from build123d import *

# Parameters (mm, degrees)
PROFILE_SKETCH_W               = 6
PROFILE_SKETCH_H               = 1
PROFILE_EXTRUDE_DEPTH          = 40
FIDUCIAL_CUT_DEPTH             = 44.409509652
FIDUCIAL_1_INDICATOR_SKETCH_W  = 2
FIDUCIAL_1_INDICATOR_SKETCH_H  = 2
FIDUCIAL_1_INDICATOR_CUT_DEPTH = 44.409509652


with BuildPart() as part:
    # Profile Sketch → Profile Extrude (new body)
    with BuildSketch(Plane(origin=(-13.83405858, 0, -105.75669297), x_dir=(-1, 0, 0), z_dir=(0, 1, 0))):
        with Locations((0, 0.5)):
            Rectangle(PROFILE_SKETCH_W, PROFILE_SKETCH_H)
    extrude(amount=PROFILE_EXTRUDE_DEPTH)

    # Fiducial Sketch → Fiducial Cut (cut, through all)
    with BuildSketch(Plane.XY.offset(-104.75669297)):
        Polygon((-12.669845017, 2), (-14.08405858, 3.414213562), (-15.498272142, 2), (-14.08405858, 0.585786438), align=None)
    fiducial_cut = extrude(amount=-FIDUCIAL_CUT_DEPTH, mode=Mode.SUBTRACT)

    # Fiducial Mirror: Fiducial Cut across plane
    add(fiducial_cut.mirror(Plane(origin=(0, 20, 0), x_dir=(0, 0, 1), z_dir=(0, -1, 0))), mode=Mode.SUBTRACT)

    # Fiducial 1 Indicator Sketch → Fiducial 1 Indicator Cut (cut, through all)
    with BuildSketch(Plane.XY.offset(-104.75669297)):
        with Locations((-14.08405858, 6)):
            Rectangle(FIDUCIAL_1_INDICATOR_SKETCH_W, FIDUCIAL_1_INDICATOR_SKETCH_H)
    extrude(amount=-FIDUCIAL_1_INDICATOR_CUT_DEPTH, mode=Mode.SUBTRACT)


solid = part.part
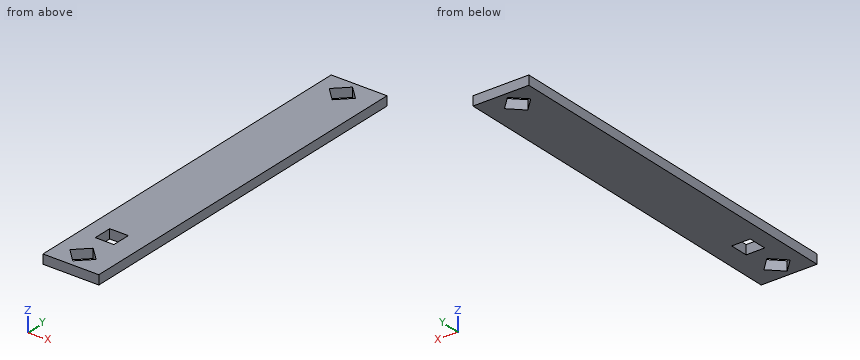
For this review, take the finished solid that the model builds, in its own axes (mm). Give positions to 0.01 mm unless a question says otherwise; leave off trailing zeros. Loops run counter-clockwise (first coordinate to the right, second up) from the corner with the lowest first, then second, coordinate; pieces in that order, holes last. Notation, with made-up numbers: M 69.25,-34 L 76.25,-34 A10 cw 76.25,-30 Z; hole C 41.25,74.5 d7. An arc over 180 degrees is marked long. Answer as a JSON object with one key per item and string values. Group by question number.
Q1. Insertion check: P1, Ø0.5, axis at x = -14, z = -105.5, coming from the -Y side. The pin has a flat end and moves straight along its axis. Give the tip position at first contact, or say it passes through.
Q2. For probe 1 along Y at (x, z) = (-14.9, -105.4); probe 2 along Y at (x, z) = (-13.6, -105.5); probe 3 along X at (y, z) = (37.5, -105.45), list the stretches that pass through material, from the lowest coordinate up. Write a range as [from, to].
Q3. Add section A-A on z = -105.2. Give the boundary of the cut face in (x, y), and give its area (3 significant figures).
Q4. Add section B-B on x = -13.7. Give the boundary of the cut face in (y, z).
Checked values:
{
 "1": {"P1": "y = 0"},
 "2": {"probe 1": "[0, 1.4], [2.6, 5], [7, 37.4], [38.6, 40]", "probe 2": "[0, 1.07], [2.93, 5], [7, 37.07], [38.93, 40]", "probe 3": "[-16.83, -15], [-13.17, -10.83]"},
 "3": {"outline": "M -16.83,0 L -10.83,0 L -10.83,40 L -16.83,40 Z; hole M -15.5,2 L -14.08,0.59 L -12.67,2 L -14.08,3.41 Z; hole M -15.5,38 L -14.08,36.59 L -12.67,38 L -14.08,39.41 Z; hole M -15.08,5 L -13.08,5 L -13.08,7 L -15.08,7 Z", "area": "228 mm²"},
 "4": {"outline": "M 0,-105.76 L 0.97,-105.76 L 0.97,-104.76 L 0,-104.76 Z; M 3.03,-105.76 L 5,-105.76 L 5,-104.76 L 3.03,-104.76 Z; M 7,-105.76 L 36.97,-105.76 L 36.97,-104.76 L 7,-104.76 Z; M 39.03,-105.76 L 40,-105.76 L 40,-104.76 L 39.03,-104.76 Z"}
}
